Check sheet for the modelled part. Datum: model origin and axes. Units: mm. Face numbers are marked on the shaded views. A direction names the side the tool comes from. Give positions to 0.01 mm unless a question says otherwise; leave off trailing zeros. Write each loop counter-clockwise with the first axis right and the second up, starting at its lowest first coordinate (ties: lowest second). Pieces come first, ordered by that corner, then holes. Notation, with made-up numbers: (29, 20) -> (82, 20) arc R29 ccw to (82, 55) -> close; hole circle Ø9 at (84.25, -18.5). An arc over 180 degrees is marked (long way). Use a Markdown table: item, result. Add a question column.
1. Scan lines: probe 1 along Y at (x, z) = (0, -3); probe 2 along Y at (x, z) = (-2, 0.5); probe 3 along Z at (x, y) = (-0.5, 27). Record each from-to range of solid material in increasing order. Write a range as [from, to].
2. Set-up check for the marked faces 1, 2, 3 and 4: record each of +Z, -Z, +X, -X, +Y, -Y from which the full face is reachable in a straight line by a thin tool's end or side.
3. Gauge pin test, flat ends, axial feed: P1, Ø2.5, axis at y = 38, z = -2.5, coming from the +X side; P2, Ø1.4, axis at x = 0, y = 63.5, coming from the -Z side; P3, Ø5, axis at x = -2, y = 40, coming from the +Z side; P4, Ø1.4, axis at y = 38, z = -2.5, coming from the -X side. Record the tip position at first contact, or that the pin passes through.
4. Cross-section at C-C (z = -3). Enter the section's corners in (x, y).
5. Cross-section at A-A (y = 25.4). Enter the section's corners in (x, z).
6. Cross-section at D-D (x = -6.5). Enter the section's corners in (y, z).
7. Cross-section at B-B (x = 0). Enter the section's corners in (y, z), then the cut area to 3 significant figures.
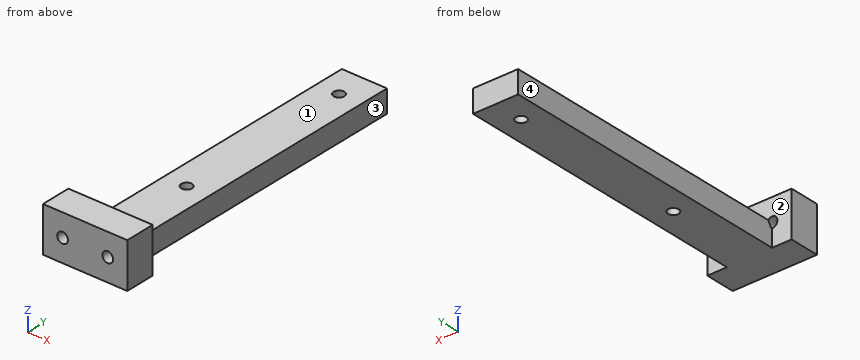
from build123d import *

# Parameters (mm, degrees)
SKETCH1_W                 = 17.78
SKETCH1_H                 = 9.525
BOSS_EXTRUDE1_DEPTH       = 69.85
SKETCH2_W                 = 17.78
SKETCH2_H                 = 4.7625
CUT_EXTRUDE1_DEPTH        = 63.5
F_4_40_TAPPED_HOLE1_D     = 2.2606
F_4_40_TAPPED_HOLE1_DEPTH = 6.604
F_4_40_TAPPED_HOLE1_TIP   = 0.679152758
F_4_40_TAPPED_HOLE2_D     = 2.2606
F_4_40_TAPPED_HOLE2_DEPTH = 8.89
F_4_40_TAPPED_HOLE2_TIP   = 0.679152758
SKETCH9_W                 = 4.1275
SKETCH9_H                 = 63.5
CUT_EXTRUDE2_DEPTH        = 71.574329655


with BuildPart() as part:
    # Sketch1 → Boss-Extrude1 (new body)
    with BuildSketch(Plane(origin=(0, 0, 0), x_dir=(1, 0, 0), z_dir=(0, 1, 0))):
        Rectangle(SKETCH1_W, SKETCH1_H)
    extrude(amount=BOSS_EXTRUDE1_DEPTH)

    # Sketch2 → Cut-Extrude1 (cut)
    with BuildSketch(Plane(origin=(0, 69.85, 0), x_dir=(1, 0, 0), z_dir=(0, 1, 0))):
        with Locations((0, -2.38125)):
            Rectangle(SKETCH2_W, SKETCH2_H)
    extrude(amount=-CUT_EXTRUDE1_DEPTH, mode=Mode.SUBTRACT)

    # #4-40 Tapped Hole1
    with Locations(Plane(origin=(0, 0, 0), x_dir=(-1, 0, 0), z_dir=(0, -1, 0))):
        with Locations((-4.7625, 0), (4.7625, 0)):
            Hole(F_4_40_TAPPED_HOLE1_D / 2, depth=F_4_40_TAPPED_HOLE1_DEPTH)
            with Locations((0, 0, -(F_4_40_TAPPED_HOLE1_DEPTH + F_4_40_TAPPED_HOLE1_TIP / 2))):  # 118° drill point
                Cone(0, F_4_40_TAPPED_HOLE1_D / 2, F_4_40_TAPPED_HOLE1_TIP, mode=Mode.SUBTRACT)

    # #4-40 Tapped Hole2
    with Locations(Plane.XY):
        with Locations((0, 25.4), (0, 63.5)):
            Hole(F_4_40_TAPPED_HOLE2_D / 2, depth=F_4_40_TAPPED_HOLE2_DEPTH)
            with Locations((0, 0, -(F_4_40_TAPPED_HOLE2_DEPTH + F_4_40_TAPPED_HOLE2_TIP / 2))):  # 118° drill point
                Cone(0, F_4_40_TAPPED_HOLE2_D / 2, F_4_40_TAPPED_HOLE2_TIP, mode=Mode.SUBTRACT)

    # Sketch9 → Cut-Extrude2 (cut, through all)
    with BuildSketch(Plane.XY):
        with Locations((-6.82625, 38.1)):
            Rectangle(SKETCH9_W, SKETCH9_H)
        with Locations((6.82625, 38.1)):
            Rectangle(SKETCH9_W, SKETCH9_H)
    extrude(amount=-CUT_EXTRUDE2_DEPTH, mode=Mode.SUBTRACT)


solid = part.part
Worked answers:
| question | item | result |
|---|---|---|
| 1 | probe 1 | y = [0, 24.27], [26.53, 62.37], [64.63, 69.85] |
| 1 | probe 2 | y = [0, 6.35] |
| 1 | probe 3 | z = [-4.76, 0] |
| 2 | face 1 | +Z, +X, -X, +Y |
| 2 | face 2 | +Z, +Y |
| 2 | face 3 | +Z, -Z, +X, +Y |
| 2 | face 4 | +Z, -Z, -X, +Y |
| 3 | P1 | stops at x = 4.76 |
| 3 | P2 | passes through |
| 3 | P3 | stops at z = 0 |
| 3 | P4 | stops at x = -4.76 |
| 4 | outline | (-8.89, 0) -> (8.89, 0) -> (8.89, 6.35) -> (4.76, 6.35) -> (4.76, 69.85) -> (-4.76, 69.85) -> (-4.76, 6.35) -> (-8.89, 6.35) -> close; hole circle Ø2.26 at (0, 25.4); hole circle Ø2.26 at (0, 63.5) |
| 5 | outline | (-4.76, -4.76) -> (-1.13, -4.76) -> (-1.13, 0) -> (-4.76, 0) -> close; (1.13, -4.76) -> (4.76, -4.76) -> (4.76, 0) -> (1.13, 0) -> close |
| 6 | outline | (0, -4.76) -> (6.35, -4.76) -> (6.35, 4.76) -> (0, 4.76) -> close |
| 7 | outline | (0, -4.76) -> (24.27, -4.76) -> (24.27, 0) -> (6.35, 0) -> (6.35, 4.76) -> (0, 4.76) -> close; (26.53, -4.76) -> (62.37, -4.76) -> (62.37, 0) -> (26.53, 0) -> close; (64.63, -4.76) -> (69.85, -4.76) -> (69.85, 0) -> (64.63, 0) -> close |
| 7 | area | 341 mm² |
